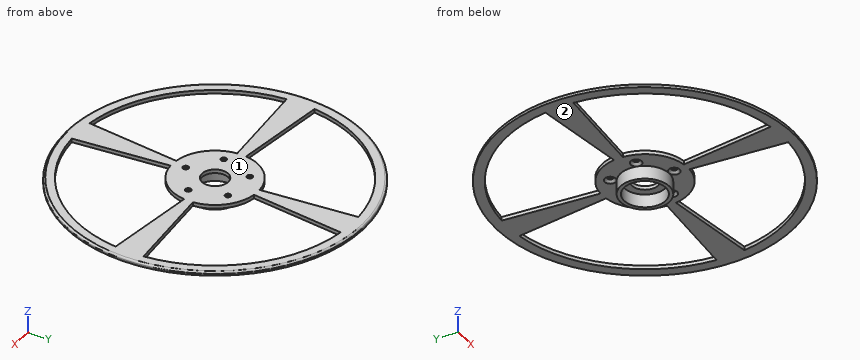
from build123d import *

# Parameters (mm, degrees)
SKETCH005_R           = 79.121
PAD_DEPTH             = 2
SKETCH010_R           = 13.0462
PAD001_DEPTH          = 7
SKETCH007_R           = 11.05
POCKET005_DEPTH       = 7
SKETCH006_R           = 7
POCKET006_DEPTH       = 5.0038
SKETCH008_R           = 1.55
POCKET007_DEPTH       = 5.0038
POLARPATTERN002_COUNT = 5
CHAMFER001_SIZE       = 1.4
POCKET008_DEPTH       = 5.0038
POLARPATTERN003_COUNT = 4
FILLET_R              = 0.999998


with BuildPart() as part:
    # Sketch005 → Pad (new body)
    with BuildSketch(Plane.XY):
        Circle(SKETCH005_R)
    extrude(amount=PAD_DEPTH)

    # Sketch010 (on Face2 of Pad) → Pad001 (join)
    with BuildSketch(Plane(origin=(0, 0, 0), x_dir=(1, 0, 0), z_dir=(0, 0, -1))):
        Circle(SKETCH010_R)
    extrude(amount=PAD001_DEPTH)

    # Sketch007 (on Face5 of Pad001) → Pocket005 (cut)
    with BuildSketch(Plane(origin=(0, 0, -7), x_dir=(1, 0, 0), z_dir=(0, 0, -1))):
        Circle(SKETCH007_R)
    extrude(amount=-POCKET005_DEPTH, mode=Mode.SUBTRACT)

    with BuildSketch(Plane(origin=(0, 0, 0), x_dir=(1, 0, 0), z_dir=(0, 0, -1))):
        Circle(SKETCH006_R)
    extrude(amount=-POCKET006_DEPTH, mode=Mode.SUBTRACT)

    # Sketch008 (on Face4 of Pocket002) → Pocket007 (cut)
    with BuildSketch(Plane(origin=(0, 0, 0), x_dir=(1, 0, 0), z_dir=(0, 0, -1))):
        with Locations((0, 16)):
            Circle(SKETCH008_R)
    pocket007 = extrude(amount=-POCKET007_DEPTH, mode=Mode.SUBTRACT)

    # PolarPattern002: Pocket007 ×5 about axis
    polarpattern002_axis = Axis((0, 0, 0), (0, 0, -1))
    for i in range(1, POLARPATTERN002_COUNT):
        add(pocket007.rotate(polarpattern002_axis, i * 360 / POLARPATTERN002_COUNT), mode=Mode.SUBTRACT)

    # Chamfer001
    chamfer001_edges = [part.edges().sort_by_distance(p)[0] for p in [
        (-1.55, -16, 0),
        (14.737928, -6.41841, 0),
        (-15.695881, -3.470134, 0),
        (-8.150588, 13.855339, 0),
        (10.65854, 12.033205, 0),
    ]]
    chamfer(chamfer001_edges, length=CHAMFER001_SIZE)

    # Sketch009 (on Face1 of Chamfer) → Pocket008 (cut)
    with BuildSketch(Plane(origin=(0, 0, 0), x_dir=(1, 0, 0), z_dir=(0, 0, -1))):
        with BuildLine():
            ThreePointArc((-2.406307, 22.733), (-16.164461, 16.164461), (-22.733, 2.406307))
            Line((-22.733, 2.406307), (-73.264802, 7.62))
            ThreePointArc((-7.62, 73.264802), (-52.085486, 52.085486), (-73.264802, 7.62))
            Line((-2.406307, 22.733), (-7.62, 73.264802))
        make_face()
    pocket008 = extrude(amount=-POCKET008_DEPTH, mode=Mode.SUBTRACT)

    # PolarPattern003: Pocket008 ×4 about axis
    polarpattern003_axis = Axis((0, 0, 0), (0, 0, -1))
    for i in range(1, POLARPATTERN003_COUNT):
        add(pocket008.rotate(polarpattern003_axis, i * 360 / POLARPATTERN003_COUNT), mode=Mode.SUBTRACT)

    # Fillet
    fillet_edges = [part.edges().sort_by_distance(p)[0] for p in [
        (-79.121, 0, 2),
    ]]
    fillet(fillet_edges, radius=FILLET_R)


solid = part.part
Geometry: final body of the model. Coordinates: model frame, mm. Face numbers are marked on the shaded views. A direction names the side the tool comes from. Give positions to 0.01 mm unless a question says otherwise; leave off trailing zeros. Loops run counter-clockwise (first coordinate to the right, second up) from the corner with the lowest first, then second, coordinate; pieces in that order, holes last. Notation, with made-up numbers: (-8, 63.25) - (28, 63.25) arc R26 cw to (28, 77.25) - close; hole circle Ø4 at (1, 74.25). An arc over 180 degrees is marked (long way). Answer as CSV lines item,"result". Start each with the question number.
1. Pin query (flat end, axial travel): P1, Ø3, axis at y = 60.5, z = 0.5, coming from the +X side; P2, Ø1.5, axis at x = -55.5, z = 0, coming from the -Y side; P3, Ø5, axis at x = -9.4, y = 12.94, coming from the -Z side. Return the tip coordinate at first contact, or that it passes through.
2. Section A-A, the plane y = 0. Return loops of the section in (x, z).
3. Section C-C, the plane y = 46. Give the number of separate pieces and of enclosed holes in the cut face, plus the area to 3 significant figures.
4. Reachability of the marked faces 1 and 2 from +Z, -Z, +X, -X, +Y, -Y: full face, straight path, thin tool, end or side. Return the list, or none.
5. Ray query, L1, parallel to X at y = -20.5, z = 1.5; L2, parallel to Y at x = 0, z = -4.75; L3, parallel to X at y = -16, z = 1.5. Return the intervals inside material, ascending.
6. Section B-B, the plane z = -4. Return loops of the section in (x, y).
Answers:
1,P1,"stops at x = 52.72"
1,P2,"stops at y = -57.12"
1,P3,"stops at z = 0.44"
2,outline,"(-79.12, 0) - (-13.05, 0) - (-13.05, -7) - (-11.05, -7) - (-11.05, 0) - (-7, 0) - (-7, 2) - (-78.12, 2) arc R1 ccw to (-79.12, 1) - close; (7, 0) - (11.05, 0) - (11.05, -7) - (13.05, -7) - (13.05, 0) - (79.12, 0) - (79.12, 1) arc R1 ccw to (78.12, 2) - (7, 2) - close"
3,separate pieces,"3"
3,enclosed holes,"0"
3,area,"46.1 mm2"
4,face 1,"+Z, +X, -X, +Y, -Y"
4,face 2,"-Z"
5,L1,"x = -76.28 to -70.75, -10.12 to 10.12, 70.75 to 76.28"
5,L2,"y = -13.05 to -11.05, 11.05 to 13.05"
5,L3,"x = -77.35 to -71.9, -16.33 to -1.55, 1.55 to 16.33, 71.9 to 77.35"
6,outline,"circle Ø26.09 at (0, 0); hole circle Ø22.1 at (0, 0)"
